Could you check a few things on this model? Use its own coordinates, in mm. A direction names the side the tool comes from. Round coordinates to 2 decimals unless told otherwise and drop trailing zeros. Write each loop counter-clockwise with the first axis right and the second up, starting at its lowest first coordinate (ties: lowest second). Pieces come first, ordered by that corner, then holes.
```python
from build123d import *

# Parameters (mm, degrees)
F0_R      = 15.24
F1_DEPTH  = 12.7
F2_R      = 15.24
F2_R_2    = 13.2588
F3_DEPTH  = 8.89
F5_DEPTH  = 7.62
F6_W      = 4.4506016257
F6_H      = 3.81
F7_DEPTH  = 25.4
F8_W      = 3.7988447554
F8_H      = 3.81
F9_DEPTH  = 25.4
F10_R     = 2.54
F11_DEPTH = 5.08
F12_DEPTH = 5.08


with BuildPart() as f1:
    # F0 (on Top) → F1 (new body)
    with BuildSketch(Plane.XY):
        Circle(F0_R)
    extrude(amount=F1_DEPTH)

    # F2 (on face) → F3 (cut)
    with BuildSketch(Plane.XY.offset(12.7)):
        Circle(F2_R)
        Circle(F2_R_2, mode=Mode.SUBTRACT)
    extrude(amount=-F3_DEPTH, mode=Mode.SUBTRACT)

    # F4 (on face) → F5 (cut)
    with BuildSketch(Plane.XY.offset(12.7)):
        with BuildLine():
            Line((13.1291263807, -1.849815645), (13.2588, -1.849815645))
            Line((13.2588, -1.849815645), (13.2588, 0))
            ThreePointArc((13.2588, 0), (13.2263418657, -0.9271775946), (13.1291263807, -1.849815645))
        make_face()
        with BuildLine():
            Line((-13.2588, -1.849815645), (-13.1291263807, -1.849815645))
            ThreePointArc((-13.1291263807, -1.849815645), (-13.2263418657, -0.9271775946), (-13.2588, 0))
            Line((-13.2588, 0), (-13.2588, -1.849815645))
        make_face()
        with BuildLine():
            ThreePointArc((13.1131024069, 1.960184355), (13.2223254315, 0.9827958199), (13.2588, 0))
            Line((13.2588, 0), (13.2588, 1.960184355))
            Line((13.2588, 1.960184355), (13.1131024069, 1.960184355))
        make_face()
        with BuildLine():
            Line((-13.2588, 1.960184355), (-13.2588, 0))
            ThreePointArc((-13.2588, 0), (-13.2223254315, 0.9827958199), (-13.1131024069, 1.960184355))
            Line((-13.1131024069, 1.960184355), (-13.2588, 1.960184355))
        make_face()
        with BuildLine():
            Line((-13.2588, 0), (13.2588, 0))
            ThreePointArc((13.2588, 0), (13.2223254315, 0.9827958199), (13.1131024069, 1.960184355))
            Line((13.1131024069, 1.960184355), (-13.1131024069, 1.960184355))
            ThreePointArc((-13.1131024069, 1.960184355), (-13.2223254315, 0.9827958199), (-13.2588, 0))
        make_face()
        with BuildLine():
            Line((-13.1291263807, -1.849815645), (13.1291263807, -1.849815645))
            ThreePointArc((13.1291263807, -1.849815645), (13.2263418657, -0.9271775946), (13.2588, 0))
            Line((13.2588, 0), (-13.2588, 0))
            ThreePointArc((-13.2588, 0), (-13.2263418657, -0.9271775946), (-13.1291263807, -1.849815645))
        make_face()
    extrude(amount=-F5_DEPTH, mode=Mode.SUBTRACT)

    # F6 (on face) → F7 (cut)
    with BuildSketch(Plane(origin=(0, -1.849815645, 0), x_dir=(-1, 0, 0), z_dir=(0, 1, 0))):
        with Locations((-10.9038255678, 6.985)):
            Rectangle(F6_W, F6_H)
    extrude(amount=-F7_DEPTH, mode=Mode.SUBTRACT)

    # F8 (on face) → F9 (cut)
    with BuildSketch(Plane.XZ.offset(-1.960184355)):
        with Locations((-11.2136800292, 6.985)):
            Rectangle(F8_W, F8_H)
    extrude(amount=-F9_DEPTH, mode=Mode.SUBTRACT)

    # F10
    f10_edges = [f1.edges().sort_by_distance(p)[0] for p in [
        (-15.24, 0, 0),
    ]]
    fillet(f10_edges, radius=F10_R)

    # F11 (cut): a face of the model
    f11_faces = [f1.faces().sort_by_distance(p)[0] for p in [
        (-9.3142576516, 5.6981527388, 6.985),
    ]]
    extrude(f11_faces, amount=-F11_DEPTH, mode=Mode.SUBTRACT)

    # F12 (cut): a face of the model
    f12_faces = [f1.faces().sort_by_distance(p)[0] for p in [
        (8.6785247549, -5.9368681555, 6.985),
    ]]
    extrude(f12_faces, amount=-F12_DEPTH, mode=Mode.SUBTRACT)


solid = f1.part
```
Q1. If I drill on L1, parallel to Z at x = -10.5, y = 5; L2, parallel to Y at x = 7, z = 1.25; L3, parallel to Y at x = -10, z = 9.5, over which ranges is the centre line in solid material (lowest first)?
Q2. Imagine slicing it at C-C, the plane y = 0. Write out the boundary of the cut face in (x, z).
Q3. I'm going to push flat-ended pins straight in: pin 1 Ø2 at (x, z) = (1.5, 2) entering from +Y; pin 2 Ø2.5 at (x, z) = (2, 8.5) entering from -Y; pin 3 Ø6 at (x, z) = (-2, 9.5) entering from +Y. Where does each tip first touch, or does it pass through?
Q4. We'd pull the mould along Y, two halves only. Please class faces 1 (the flat face through (0, -6, 12.7)), 2 (the flat face through (3.599, -6, 7)), 3 (the cylindrical face through (-3.3, -14.88, 3.17)): pulls with the +Y half, pulls with the -Y half, needs draft (parallel to the pull), parting line crosses it, or undercut.
Q5. Imagine slicing it at A-A, the plane z = 5.5. Write out the boundary of the cut face in (x, y).
Q6. On a 3-axis mill with a long thin cutter (end or side, diameter ignored), from which of +Z, -Z, +X, -X, +Y, -Y can I reach the whole of each face in a straight line? I mean faces 4 (the flat face through (-8, 6, 8.89)), 5 (the flat face through (7, -6, 8.89)), 6 (the flat face through (-1.2, -13.5, 3.81)). Say none if no direction works.
Q7. Imagine slicing it at B-B, the plane x = 0. Write out the boundary of the cut face in (y, z).
Results found:
1. L1: z = 0 to 5.08, 8.89 to 12.7
1. L2: y = -13.14 to 13.14
1. L3: y = -8.71 to -1.85, 1.96 to 8.71
2. outline: (-15.24, 2.54) arc R2.54 ccw to (-12.7, 0) - (12.7, 0) arc R2.54 ccw to (15.24, 2.54) - (15.24, 3.81) - (13.26, 3.81) - (13.26, 5.08) - (-13.26, 5.08) - (-13.26, 3.81) - (-15.24, 3.81) - close
3. pin 1: stops at y = 15.23
3. pin 2: stops at y = -13.24
3. pin 3: stops at y = 13.26
4. face 1: needs draft
4. face 2: undercut
4. face 3: parting line crosses it
5. outline: (-13.13, -1.85) arc R13.26 ccw to (8.68, -10.02) - (3.6, -10.02) - (3.6, -1.85) - close; (-9.31, 9.44) - (-4.23, 9.44) - (-4.23, 1.96) - (13.11, 1.96) arc R13.26 ccw to start
6. face 4: -X
6. face 5: +X
6. face 6: +Z
7. outline: (-15.24, 2.54) arc R2.54 ccw to (-12.7, 0) - (12.7, 0) arc R2.54 ccw to (15.24, 2.54) - (15.24, 3.81) - (13.26, 3.81) - (13.26, 12.7) - (1.96, 12.7) - (1.96, 5.08) - (-1.85, 5.08) - (-1.85, 12.7) - (-13.26, 12.7) - (-13.26, 3.81) - (-15.24, 3.81) - close
